Can you work these out from the drawing? Everything is in mm from the part's minimum corner. A direction names the side the tool comes from. Give positions to 0.01 mm unless a question says otherwise; leave off trailing zeros. Write each loop counter-clockwise with the first axis right and the second up, starting at its lowest first coordinate (ties: lowest second). Pieces come first, ordered by that corner, then holes. Notation, with made-up numbers: (40, 70.5) -> (86, 70.5) arc R36 cw to (86, 107.5) -> close; hole circle Ø9 at (-2.75, -9). An arc over 180 degrees is marked (long way). Use one line per item in the form item = value.
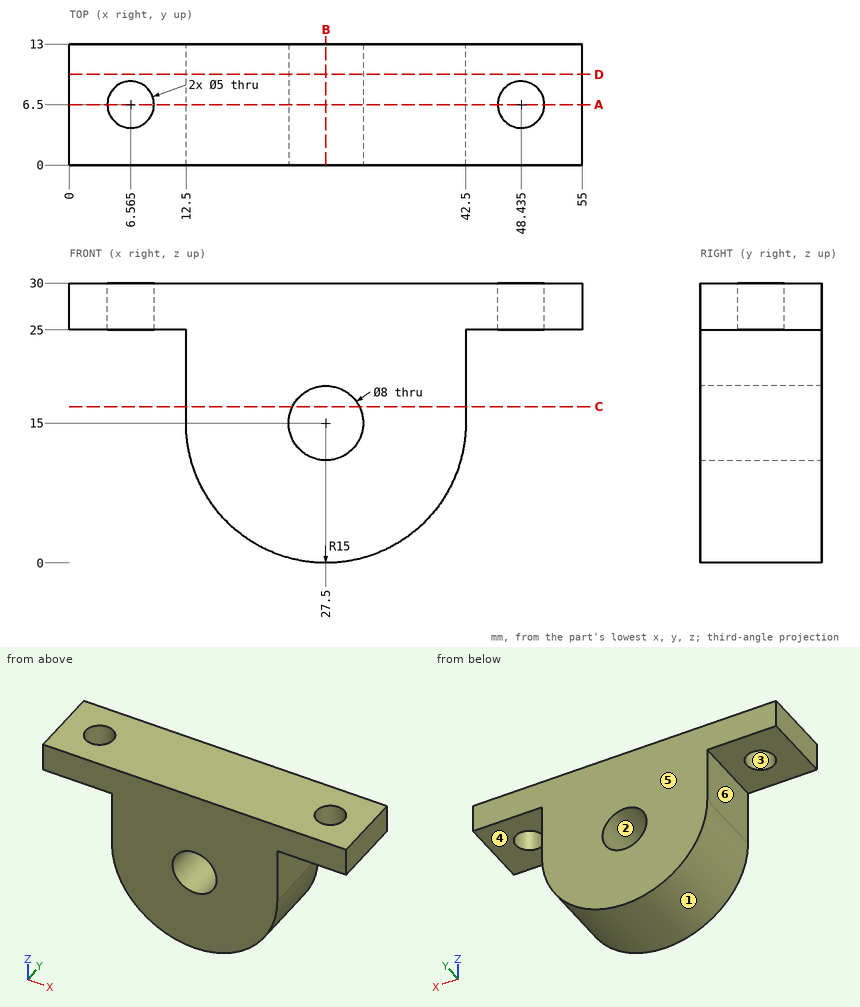
Q1. If we mould it in two halves opening along Z, with no side actions, what happens to the marked faces 1, 2 and 3? For each: +Z half, -Z half, draft (parallel to the pull), parting line (faces both ways), or undercut.
Result set:
face_1 = -Z half
face_2 = undercut
face_3 = draft
Q2. Which directions (+Z, -Z, +X, -X, +Y, -Y) give clear straight access to the entire face, cutting with the end or side of a thin tool? Please do the marked faces 4, 5 and 6.
Result set:
face_4 = -Z, +X, +Y, -Y
face_5 = +Z, -Z, +X, -X, +Y
face_6 = -Z, -X, +Y, -Y
Q3. I want a section at B-B, the plane x = 27.5. Write out the boundary of the cut face in (y, z).
Result set:
outline = (0, 0) -> (13, 0) -> (13, 11) -> (0, 11) -> close; (0, 19) -> (13, 19) -> (13, 30) -> (0, 30) -> close
Q4. Will these pins go through, and if not, where does the flat tip stop? pin 1 Ø1.5 at (y, z) = (1.5, 12) entering from -X; pin 2 Ø6 at (y, z) = (5.5, 16) entering from -X; pin 3 Ø6 at (y, z) = (4.5, 6) entering from +X.
Result set:
pin_1 = 12.67
pin_2 = 12.5
pin_3 = 41.25
Q5. If I drill on line 1 along Z through (x, y) = (27.5, 9.5); line 2 along X through (y, z) = (6.5, 15); line 3 along X through (y, z) = (3, 24), over which ranges is the centre line in solid material (lowest first)? Write a range as from..to.
Result set:
line_1 = 0..11, 19..30
line_2 = 12.5..23.5, 31.5..42.5
line_3 = 12.5..42.5
Q6. I want a section at C-C, the plane z = 16.75. Write out the boundary of the cut face in (x, y).
Result set:
outline = (12.5, 0) -> (23.9, 0) -> (23.9, 13) -> (12.5, 13) -> close; (31.1, 0) -> (42.5, 0) -> (42.5, 13) -> (31.1, 13) -> close
Q7. I want a section at A-A, the plane y = 6.5. Write out the boundary of the cut face in (x, z) (3 decimals).
Result set:
outline = (0, 25) -> (4.065, 25) -> (4.065, 30) -> (0, 30) -> close; (9.065, 25) -> (12.5, 25) -> (12.5, 15) arc R15 ccw to (42.5, 15) -> (42.5, 25) -> (45.935, 25) -> (45.935, 30) -> (9.065, 30) -> close; (50.935, 25) -> (55, 25) -> (55, 30) -> (50.935, 30) -> close; hole circle Ø8 at (27.5, 15)
Q8. I want a section at D-D, the plane y = 9.75. Write out the boundary of the cut face in (x, z), and give its area (3 significant figures).
Result set:
outline = (0, 25) -> (12.5, 25) -> (12.5, 15) arc R15 ccw to (42.5, 15) -> (42.5, 25) -> (55, 25) -> (55, 30) -> (0, 30) -> close; hole circle Ø8 at (27.5, 15)
area = 878 mm2
